Input: part model. Units: mm. Frame: model coordinates. Coordinates: 2 decimals unless noted, no trailing zeros. Loops run counter-clockwise (first coordinate to the right, second up) from the corner with the lowest first, then second, coordinate; pieces in that order, holes last.
(1) Section A-A, the plane y = -9.25. Return loops of the section in (x, z).
(2) Line query: L1, parallel to X at y = -5, z = 0; L2, parallel to Z at x = 0.25, y = -7.5; L3, parallel to X at y = 4.25, z = 0.25. Output: solid intervals per line, ascending.
(3) Contact query for flat-ended pins moving along their axis: P1, Ø1, axis at x = 0, y = 3, coming from the -Z side; P2, Ø6, axis at x = 0.5, y = -6.5, coming from the +Z side; P3, Ø5, axis at y = -9, z = -3, coming from the -X side. Output: stop coordinate, or through.
(4) Mould query, pull axis Y, two halves, no side actions, for faces 1 (the face through (-3.417, -8.381, 0.759)), 2 (the face through (2.2, 1, 1)), 3 (the face through (-2.3, -17, -0.7)). Classes: released by +Y, released by -Y, zero draft, split by the parting line, or undercut.
```python
from build123d import *

# Parameters (mm, degrees)
SKETCH_2_R          = 3.5
EXTRUDE_1_DEPTH     = 17
SKETCH_3_R          = 2.25
CUT_EXTRUDE_1_DEPTH = 18


with BuildPart() as part:
    # 草图1 → 旋转1 (revolve)
    with BuildSketch(Plane.XY):
        with BuildLine():
            Line((0, 0), (0, 1))
            Line((0, 1), (4.713145709, 1))
            ThreePointArc((4.713145709, 1), (3.295495491, 6.508537741), (0, 11.144638437))
            Line((0, 11.144638437), (0, 12.5))
            ThreePointArc((0, 12.5), (4.228807467, 6.872751435), (5.75, 0))
            Line((5.75, 0), (0, 0))
        make_face()
    revolve(axis=Axis((0, 11.144638437, 0), (0, 1, 0)))

    # 草图2 → 凸台-拉伸1 (add)
    with BuildSketch(Plane.XZ):
        with Locations(Location((0, 0, 0), (0, 0, 270))):
            Circle(SKETCH_2_R)
    extrude(amount=EXTRUDE_1_DEPTH)

    # 草图3 → 切除-拉伸1 (cut)
    with BuildSketch(Plane.XZ.offset(17)):
        with Locations(Location((0, 0, 0), (0, 0, 270))):
            Circle(SKETCH_3_R)
    extrude(amount=-CUT_EXTRUDE_1_DEPTH, mode=Mode.SUBTRACT)


solid = part.part
```
Report:
1. outline: circle Ø7 at (0, 0); hole circle Ø4.5 at (0, 0)
2. L1: x = -3.5 to -2.25, 2.25 to 3.5
2. L2: z = -3.49 to -2.24, 2.24 to 3.49
2. L3: x = -5.17 to -4.13, 4.13 to 5.17
3. P1: stops at z = -5.55
3. P2: stops at z = 3.5
3. P3: stops at x = -3.46
4. face 1: zero draft
4. face 2: undercut
4. face 3: released by -Y
